```python
from build123d import *

# Parameters (mm, degrees)
SKETCH_1_W               = 900
SKETCH_1_H               = 2100
SKETCH_1_W_2             = 810
SKETCH_1_H_2             = 2000
EXTRUDE_1_DEPTH          = 100
SKETCH_2_W               = 20
SKETCH_2_H               = 100
EXTRUDE_2_DEPTH          = 30
SKETCH_3_R               = 20
EXTRUDE_3_DEPTH          = 100
PATTERN_LINEAR_1_COUNT   = 2
PATTERN_LINEAR_1_PITCH   = 1200
MIRROR_1_COPY_1_SKETCH_W = 20
MIRROR_1_COPY_1_SKETCH_H = 100
MIRROR_1_COPY_1_DEPTH    = 30
MIRROR_1_COPY_2_SKETCH_R = 20
MIRROR_1_COPY_2_DEPTH    = 100
DELETE_FACE_1_OUTLINE_W  = 41
DELETE_FACE_1_OUTLINE_H  = 100
DELETE_FACE_1_DEPTH      = 50


# Read off the part's stored shape, not the designer's step: Удалить грань1
with BuildPart() as part:
    # Эскиз1 → Бобышка-Вытянуть1 (new body)
    with BuildSketch(Plane.XY):
        with Locations((450, 1050)):
            Rectangle(SKETCH_1_W, SKETCH_1_H)
        with Locations((450, 1050)):
            Rectangle(SKETCH_1_W_2, SKETCH_1_H_2, mode=Mode.SUBTRACT)
    extrude(amount=-EXTRUDE_1_DEPTH)

    # Эскиз2 → Бобышка-Вытянуть2 (add)
    with BuildSketch(Plane.XY):
        with Locations((865, 1600)):
            Rectangle(SKETCH_2_W, SKETCH_2_H)
    extrude_2 = extrude(amount=EXTRUDE_2_DEPTH)

    # Эскиз3 → Бобышка-Вытянуть3 (add)
    with BuildSketch(Plane(origin=(0, 1650, 0), x_dir=(1, 0, 0), z_dir=(0, 1, 0))):
        with Locations((855, -30)):
            Circle(SKETCH_3_R)
    extrude_3 = extrude(amount=-EXTRUDE_3_DEPTH)

    # Линейный массив1: Бобышка-Вытянуть2, Бобышка-Вытянуть3 ×2
    with Locations(*[(0, -i * PATTERN_LINEAR_1_PITCH, 0) for i in range(1, PATTERN_LINEAR_1_COUNT)]):
        add(extrude_2)
        add(extrude_3)

    # Зеркальное отражение1: Бобышка-Вытянуть2, Бобышка-Вытянуть3 across plane
    add(extrude_2.mirror(Plane.XY.offset(-50)))
    add(extrude_3.mirror(Plane.XY.offset(-50)))

    # Зеркальное отражение1 copy 1 sketch → Зеркальное отражение1 copy 1 (add)
    with BuildSketch(Plane(origin=(0, -1200, -100), x_dir=(1, 0, 0), z_dir=(0, 0, -1))):
        with Locations((865, -1600)):
            Rectangle(MIRROR_1_COPY_1_SKETCH_W, MIRROR_1_COPY_1_SKETCH_H)
    extrude(amount=MIRROR_1_COPY_1_DEPTH)

    # Зеркальное отражение1 copy 2 sketch → Зеркальное отражение1 copy 2 (add)
    with BuildSketch(Plane(origin=(0, 450, -100), x_dir=(1, 0, 0), z_dir=(0, 1, 0))):
        with Locations((855, 30)):
            Circle(MIRROR_1_COPY_2_SKETCH_R)
    extrude(amount=-MIRROR_1_COPY_2_DEPTH)

    # Delete Face 1 outline → Delete Face 1 (cut)
    with BuildSketch(Plane.XY):
        with Locations((854.5, 1600)):
            Rectangle(DELETE_FACE_1_OUTLINE_W, DELETE_FACE_1_OUTLINE_H)
        with Locations((854.5, 400)):
            Rectangle(DELETE_FACE_1_OUTLINE_W, DELETE_FACE_1_OUTLINE_H)
    extrude(amount=DELETE_FACE_1_DEPTH, mode=Mode.SUBTRACT)


with BuildPart() as body_2:
    # Зеркальное отражение2: mirrored copy
    add(part.part.mirror(Plane(origin=(0, 0, 0), x_dir=(0, 0, 1), z_dir=(1, 0, 0))))


solid = body_2.part
```
CAD build for the part. Positions are in the model's coordinates, mm. A direction names the side the tool comes from. Coordinates: 2 decimals unless noted, no trailing zeros. Write each loop counter-clockwise with the first axis right and the second up, starting at its lowest first coordinate (ties: lowest second). Pieces come first, ordered by that corner, then holes.
(1) Cut at B-B, the plane x = -180. List the corners of the cut face in (y, z), and give its area (3 significant figures).
(2) Flat gauge pins, fed straight in: pin 1 (10 mm diameter, centred on y = 751.5, z = -108, fed in from +X); pin 2 (10 mm diameter, centred on y = 600, z = -53.5, fed in from +X); pin 3 (15 mm diameter, centred on y = 1615.5, z = -113, fed in from -X); pin 4 (12 mm diameter, centred on x = -863, z = -127, fed in from +Y). Where does each tip first touch, or does it go through?
(3) Drill centre lines: probe 1 along Y at (x, z) = (-438.5, -45); probe 2 along X at (y, z) = (1228, -57). Where is each one in solid material? Low to high.
(4) Cut at C-C, the plane z = -19. List the corners of the cut face in (x, y), and give its area (3 significant figures).
(5) Cut at A-A, the plane y = 1364. List the corners of the cut face in (x, z), and give its area (3 significant figures).
(6) 3-axis set-ups, long thin cutter, end or side, ignore diameter. For faces 5 (the face through (-45, 1036, -49)), 6 (the face through (-855, 1650, -125)), 7 (the face through (-855, 1550, -125)), 8 (the face through (-855, 350, -125)): which of +Z, -Z, +X, -X, +Y, -Y reach the whole face in a straight line?
(7) Two-plate mould, pull along X, no slides. Class faces 1 (the face through (-900, 1035, -49)), 2 (the face through (-855, 1036, -54)), 3 (the face through (-444, 50, -49)), 4 (the face through (-855, 450, -125)): +X half, -X half, draft (parallel to the pull), parting line (faces both ways), or undercut.
Geometry says:
1. outline: (0, -100) - (50, -100) - (50, 0) - (0, 0) - close; (2050, -100) - (2100, -100) - (2100, 0) - (2050, 0) - close
1. area: 10,000 mm2
2. pin 1: passes through
2. pin 2: stops at x = 0
2. pin 3: stops at x = -875
2. pin 4: stops at y = 1650
3. probe 1: y = 0 to 50, 2050 to 2100
3. probe 2: x = -900 to -855, -45 to 0
4. outline: (-900, 0) - (0, 0) - (0, 2100) - (-900, 2100) - close; hole (-855, 50) - (-45, 50) - (-45, 2050) - (-855, 2050) - close
4. area: 270,000 mm2
5. outline: (-900, -100) - (-855, -100) - (-855, 0) - (-900, 0) - close; (-45, -100) - (0, -100) - (0, 0) - (-45, 0) - close
5. area: 9,000 mm2
6. face 5: +Z, -Z
6. face 6: -Z, +X, -X, +Y
6. face 7: -Z, +X, -X
6. face 8: -Z, +X, -X, -Y
7. face 1: -X half
7. face 2: undercut
7. face 3: undercut
7. face 4: draft
